from build123d import *

# Parameters (mm, degrees)
SKETCH1_W               = 20
SKETCH1_H               = 46
SKETCH1_R               = 1.25
SKETCH1_R_2             = 6
SKETCH1_R_3             = 1.5
BOSS_EXTRUDE1_DEPTH     = 3
CUT_EXTRUDE1_DEPTH      = 26.258661881
CUT_EXTRUDE1_DEPTH_BACK = 26.258661881
SKETCH2_W               = 20
SKETCH2_H               = 13.653393661


with BuildPart() as part:
    # Sketch1 → Boss-Extrude1 (new body)
    with BuildSketch(Plane(origin=(0, 0, 0), x_dir=(1, 0, 0), z_dir=(0, 1, 0))):
        Rectangle(SKETCH1_W, SKETCH1_H)
        with Locations(Location((0, 18, 0), (0, 0, 270))):
            Circle(SKETCH1_R, mode=Mode.SUBTRACT)
        with Locations(Location((0, 9.5, 0), (0, 0, 270))):
            Circle(SKETCH1_R_2, mode=Mode.SUBTRACT)
        with Locations(Location((0, 1, 0), (0, 0, 90))):
            Circle(SKETCH1_R, mode=Mode.SUBTRACT)
        with Locations(Location((0, -13, 0), (0, 0, 270))):
            Circle(SKETCH1_R_3, mode=Mode.SUBTRACT)
    extrude(amount=BOSS_EXTRUDE1_DEPTH)

    # Sketch2 → Cut-Extrude1 (cut, two sides: drawn at the far end of the back side and taken through both)
    with BuildSketch(Plane(origin=(0, 3, 0), x_dir=(1, 0, 0), z_dir=(0, 1, 0)).offset(-CUT_EXTRUDE1_DEPTH_BACK)):
        with Locations((0, -29.826696831)):
            Rectangle(SKETCH2_W, SKETCH2_H)
        with BuildLine():
            ThreePointArc((10, -16.653393661), (0, -18.5), (-10, -16.653393661))
            Line((-10, -16.653393661), (-10, -23))
            Line((-10, -23), (10, -23))
            Line((10, -23), (10, -16.653393661))
        make_face()
    extrude(amount=CUT_EXTRUDE1_DEPTH + CUT_EXTRUDE1_DEPTH_BACK, mode=Mode.SUBTRACT)


solid = part.part
Can you work these out from the model? Positions are in its coordinate system, mm. Round coordinates to 2 decimals unless told otherwise and drop trailing zeros. Write each loop counter-clockwise with the first axis right and the second up, starting at its lowest first coordinate (ties: lowest second). Pieces come first, ordered by that corner, then holes. Notation, with made-up numbers: (36.25, -15.5) -> (87.25, -15.5) arc R26 ccw to (87.25, 20.5) -> close; hole circle Ø4 at (-9.75, -35.5). An arc over 180 degrees is marked (long way). Use one line per item in the form item = value. Start each with the question number.
Q1. Imagine slicing it at C-C (y = 2.1). Please give me the cut outline in (x, z).
Q2. Imagine slicing it at B-B (x = 0). Please give me the cut outline in (y, z).
Q3. We'd pull the mould along Z, two halves only. Please class faces 1 (the face through (-0.05, 1.48, 0.25)), 2 (the face through (0, 1, -23)), 3 (the face through (0.1, 1.5, 18.5)), 4 (the face through (-10, 1, -3)): +Z half, -Z half, draft (parallel to the pull), parting line (faces both ways), or undercut.
Q4. Imagine slicing it at D-D (x = -5.5). Please give me the cut outline in (y, z), then the cut area to 3 significant figures.
Q5. Imagine slicing it at A-A (z = -9.5). Please give me the cut outline in (x, y), then the cut area to 3 significant figures.
Q6. If I drill on probe 1 along X at (y, z) = (1.7, -18); probe 2 along X at (y, z) = (1.95, 13); probe 3 along Z at (x, y) = (-5, 2.5), over which ranges is the centre line in solid material (lowest first)? Write a range as [from, to].
Worked out:
q1.outline = (-10, -23) -> (10, -23) -> (10, 16.65) arc R28 ccw to (-10, 16.65) -> close; hole circle Ø12 at (0, -9.5); hole circle Ø3 at (0, 13); hole circle Ø2.5 at (0, -18); hole circle Ø2.5 at (0, -1)
q2.outline = (0, -23) -> (3, -23) -> (3, -19.25) -> (0, -19.25) -> close; (0, -16.75) -> (3, -16.75) -> (3, -15.5) -> (0, -15.5) -> close; (0, -3.5) -> (3, -3.5) -> (3, -2.25) -> (0, -2.25) -> close; (0, 0.25) -> (3, 0.25) -> (3, 11.5) -> (0, 11.5) -> close; (0, 14.5) -> (3, 14.5) -> (3, 18.5) -> (0, 18.5) -> close
q3.face_1 = undercut
q3.face_2 = -Z half
q3.face_3 = +Z half
q3.face_4 = draft
q4.outline = (0, -23) -> (3, -23) -> (3, -11.9) -> (0, -11.9) -> close; (0, -7.1) -> (3, -7.1) -> (3, 17.95) -> (0, 17.95) -> close
q4.area = 108 mm^2
q5.outline = (-10, 0) -> (-6, 0) -> (-6, 3) -> (-10, 3) -> close; (6, 0) -> (10, 0) -> (10, 3) -> (6, 3) -> close
q5.area = 24.0 mm^2
q6.probe_1 = [-10, -1.25], [1.25, 10]
q6.probe_2 = [-10, -1.5], [1.5, 10]
q6.probe_3 = [-23, -12.82], [-6.18, 18.05]
